Check sheet for the modelled part. Datum: model origin and axes. Units: mm. A direction names the side the tool comes from. Round coordinates to 2 decimals unless told otherwise and drop trailing zeros. Order: outer loops, then holes, each group sorted by start corner. A loop starts at its lowest first (then second) coordinate and runs counter-clockwise, first axis right, second up. Notation, with made-up numbers: (-30, 2) -> (28, 2) arc R28 ccw to (28, 24) -> close; hole circle Ø4 at (-32.75, 27). An arc over 180 degrees is marked (long way). Answer in a Markdown table with one row per item.
```python
from build123d import *

# Parameters (mm, degrees)
SKETCH1_R           = 22.5
BOSS_EXTRUDE1_DEPTH = 76
SKETCH2_R           = 25
BOSS_EXTRUDE2_DEPTH = 10
SKETCH3_R           = 12.5
BOSS_EXTRUDE3_DEPTH = 4
SKETCH4_R           = 2.5
CUT_EXTRUDE1_DEPTH  = 8
CIRPATTERN1_COUNT   = 4
SKETCH5_R           = 2.5
CUT_EXTRUDE2_DEPTH  = 8
CIRPATTERN2_COUNT   = 5


with BuildPart() as part:
    # Sketch1 → Boss-Extrude1 (new body)
    with BuildSketch(Plane(origin=(0, 0, 0), x_dir=(1, 0, 0), z_dir=(0, 1, 0))):
        with Locations(Location((0, 0, 0), (0, 0, 270))):
            Circle(SKETCH1_R)
    extrude(amount=BOSS_EXTRUDE1_DEPTH)

    # Sketch2 → Boss-Extrude2 (add)
    with BuildSketch(Plane(origin=(0, 76, 0), x_dir=(1, 0, 0), z_dir=(0, 1, 0))):
        with Locations(Location((0, 0, 0), (0, 0, 270))):
            Circle(SKETCH2_R)
    extrude(amount=BOSS_EXTRUDE2_DEPTH)

    # Sketch3 → Boss-Extrude3 (add)
    with BuildSketch(Plane(origin=(0, 86, 0), x_dir=(1, 0, 0), z_dir=(0, 1, 0))):
        with Locations(Location((0, 0, 0), (0, 0, 270))):
            Circle(SKETCH3_R)
    extrude(amount=BOSS_EXTRUDE3_DEPTH)

    # Sketch4 → Cut-Extrude1 (cut)
    with BuildSketch(Plane(origin=(0, 86, 0), x_dir=(1, 0, 0), z_dir=(0, 1, 0))):
        with Locations(Location((-20, 0, 0), (0, 0, 270))):
            Circle(SKETCH4_R)
    cut_extrude1 = extrude(amount=-CUT_EXTRUDE1_DEPTH, mode=Mode.SUBTRACT)

    # CirPattern1: Cut-Extrude1 ×4 about axis
    cirpattern1_axis = Axis((0, 0, 0), (0, 1, 0))
    for i in range(1, CIRPATTERN1_COUNT):
        add(cut_extrude1.rotate(cirpattern1_axis, i * 360 / CIRPATTERN1_COUNT), mode=Mode.SUBTRACT)

    # Sketch5 → Cut-Extrude2 (cut)
    with BuildSketch(Plane.XZ):
        with Locations(Location((0, 17.5, 0), (0, 0, 270))):
            Circle(SKETCH5_R)
    cut_extrude2 = extrude(amount=-CUT_EXTRUDE2_DEPTH, mode=Mode.SUBTRACT)

    # CirPattern2: Cut-Extrude2 ×5 about axis
    cirpattern2_axis = Axis((0, 0, 0), (0, 1, 0))
    for i in range(1, CIRPATTERN2_COUNT):
        add(cut_extrude2.rotate(cirpattern2_axis, i * 360 / CIRPATTERN2_COUNT), mode=Mode.SUBTRACT)


solid = part.part
```
(1) Section check A-A on y = 81.5. Record the boundary of the cut face in (x, z), plus the area to 3 significant figures.
Solutions:
| item | result |
|---|---|
| outline | circle Ø50 at (0, 0); hole circle Ø5 at (-20, 0); hole circle Ø5 at (0, -20); hole circle Ø5 at (0, 20); hole circle Ø5 at (20, 0) |
| area | 1,880 mm^2 |
(2) Scan lines: probe 1 along X at (y, z) = (79.75, 0); probe 2 along Y at (x, z) = (12, 18); probe 3 along X at (y, z) = (5.5, 17.5). Record each from-to range of solid material in increasing order. Write a range as from..to.
Solutions:
| item | result |
|---|---|
| probe 1 | -25..-22.5, -17.5..17.5, 22.5..25 |
| probe 2 | 0..86 |
| probe 3 | -14.14..-2.5, 2.5..14.14 |
(3) Depth check by flat-ended pin: pin 1 Ø2 at (y, z) = (78, -1) entering from +X; pin 2 Ø2 at (x, y) = (-19.5, 39) entering from +Z; pin 3 Ø6 at (y, z) = (77, 17.5) entering from -X; pin 4 Ø5.5 at (x, z) = (0.5, 18.5) entering from -Y. Enter the tip coordinate at first touch or a pass-through.
Solutions:
| item | result |
|---|---|
| pin 1 | x = 25 |
| pin 2 | z = 12.81 |
| pin 3 | x = -20.37 |
| pin 4 | y = 0 |
(4) Tool access check on faces 1 (the flat face through (0, 78, 20)), 2 (the cylindrical face through (7.509, 80.93, 23.846)), 3 (the cylindrical face through (-7.814, 3.944, -14.528)). Record the directions out of +Z, -Z, +X, -X, +Y, -Y that give a thin tool (end or side, any length) a straight path to the whole face; none if there is none.
Solutions:
| item | result |
|---|---|
| face 1 | +Y |
| face 2 | +Y, -Y |
| face 3 | -Y |
(5) Section check B-B on x = 0. Record the boundary of the cut face in (y, z).
Solutions:
| item | result |
|---|---|
| outline | (0, -22.5) -> (76, -22.5) -> (76, -25) -> (86, -25) -> (86, -22.5) -> (78, -22.5) -> (78, -17.5) -> (86, -17.5) -> (86, -12.5) -> (90, -12.5) -> (90, 12.5) -> (86, 12.5) -> (86, 17.5) -> (78, 17.5) -> (78, 22.5) -> (86, 22.5) -> (86, 25) -> (76, 25) -> (76, 22.5) -> (0, 22.5) -> (0, 20) -> (8, 20) -> (8, 15) -> (0, 15) -> close |
(6) Draft check along X on faces 4 (the cylindrical face through (-8.618, 37.468, 20.784)), 5 (the cylindrical face through (0, 4, 20)), 6 (the flat face through (0, 90, 0)). Enter one of: pulls with the +X half, pulls with the -X half, needs draft (parallel to the pull), parting line crosses it, or undercut.
Solutions:
| item | result |
|---|---|
| face 4 | parting line crosses it |
| face 5 | undercut |
| face 6 | needs draft |
(7) Section check D-D on y = 30. Record the boundary of the cut face in (x, z), plus the area to 3 significant figures.
Solutions:
| item | result |
|---|---|
| outline | circle Ø45 at (0, 0) |
| area | 1,590 mm^2 |
(8) Section check C-C on z = 0. Record the boundary of the cut face in (x, y), plus the area to 3 significant figures.
Solutions:
| item | result |
|---|---|
| outline | (-25, 76) -> (-22.5, 76) -> (-22.5, 0) -> (22.5, 0) -> (22.5, 76) -> (25, 76) -> (25, 86) -> (22.5, 86) -> (22.5, 78) -> (17.5, 78) -> (17.5, 86) -> (12.5, 86) -> (12.5, 90) -> (-12.5, 90) -> (-12.5, 86) -> (-17.5, 86) -> (-17.5, 78) -> (-22.5, 78) -> (-22.5, 86) -> (-25, 86) -> close |
| area | 3,940 mm^2 |
